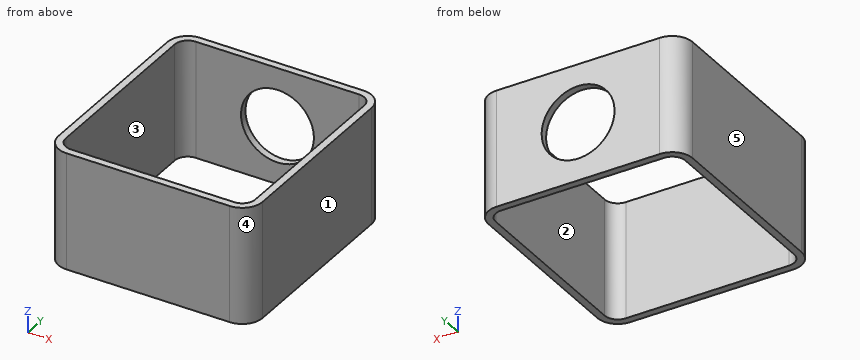
```python
from build123d import *

# Parameters (mm, degrees)
SKETCH_1_W          = 28
SKETCH_1_H          = 30
SKETCH_1_W_2        = 26
SKETCH_1_H_2        = 28
EXTRUDE_1_DEPTH     = 16
FILLET_1_R          = 1.8
FILLET_2_R          = 2.8
SKETCH_2_R          = 5
CUT_EXTRUDE_1_DEPTH = 16


with BuildPart() as part:
    # Эскиз1 → Бобышка-Вытянуть1 (new body)
    with BuildSketch(Plane.XY):
        with Locations((14, 15)):
            Rectangle(SKETCH_1_W, SKETCH_1_H)
        with Locations((14, 15)):
            Rectangle(SKETCH_1_W_2, SKETCH_1_H_2, mode=Mode.SUBTRACT)
    extrude(amount=EXTRUDE_1_DEPTH)

    # Скругление1
    fillet_1_edges = [part.edges().sort_by_distance(p)[0] for p in [
        (27, 29, 8),
        (1, 29, 8),
        (1, 1, 8),
        (27, 1, 8),
    ]]
    fillet(fillet_1_edges, radius=FILLET_1_R)

    # Скругление2
    fillet_2_edges = [part.edges().sort_by_distance(p)[0] for p in [
        (0, 30, 8),
        (28, 30, 8),
        (28, 0, 8),
        (0, 0, 8),
    ]]
    fillet(fillet_2_edges, radius=FILLET_2_R)

    # Эскиз2 → Вырез-Вытянуть1 (cut)
    with BuildSketch(Plane(origin=(0, 30, 0), x_dir=(1, 0, 0), z_dir=(0, 1, 0))):
        with Locations(Location((14, -8, 0), (0, 0, 270))):
            Circle(SKETCH_2_R)
    extrude(amount=-CUT_EXTRUDE_1_DEPTH, mode=Mode.SUBTRACT)


solid = part.part
```
Design review of the part built by this model. Coordinates are the model's own, in mm. Face numbers are marked on the shaded views. A direction names the side the tool comes from. Round coordinates to 2 decimals unless told otherwise and drop trailing zeros. Write each loop counter-clockwise with the first axis right and the second up, starting at its lowest first coordinate (ties: lowest second). Pieces come first, ordered by that corner, then holes. Notation, with made-up numbers: (-3.75, 46) -> (35.25, 46) arc R25 cw to (35.25, 62) -> close; hole circle Ø2 at (53, 23.25). An arc over 180 degrees is marked (long way). Write item = value, one per line. Start each with the question number.
1) Take a section at D-D, the plane z = 1.5. State the section outline as (x, y) points.
2) Mouldability with a two-part tool opening along X and no side actions: class the marked faces 3, 4 and 5 as +X half, -X half, draft (parallel to the pull), parting line (faces both ways), or undercut.
3) Take a section at A-A, the plane x = 10. State the section outline as (y, z) points.
4) Tool access review of the marked faces 1 and 2: name each direction out of +Z, -Z, +X, -X, +Y, -Y from which nothing blocks a thin tool from reaching the whole face with its end or side.
5) Take a section at B-B, the plane y = 8.25. State the section outline as (x, z) points, plus the area to 3 significant figures.
6) Take a section at C-C, the plane x = 6.75. State the section outline as (y, z) points.
7) Wall thickness on probe 1 along Y at (x, z) = (5, 12); probe 2 along X at (y, z) = (22, 14.75); probe 3 along X at (y, z) = (29.65, 8): over which ranges is each line inside the solid? List them lowest first. Write a range as from..to.
Results list:
q1.outline = (0, 2.8) arc R2.8 ccw to (2.8, 0) -> (25.2, 0) arc R2.8 ccw to (28, 2.8) -> (28, 27.2) arc R2.8 ccw to (25.2, 30) -> (2.8, 30) arc R2.8 ccw to (0, 27.2) -> close; hole (1, 2.8) arc R1.8 ccw to (2.8, 1) -> (25.2, 1) arc R1.8 ccw to (27, 2.8) -> (27, 27.2) arc R1.8 ccw to (25.2, 29) -> (2.8, 29) arc R1.8 ccw to (1, 27.2) -> close
q2.face_3 = undercut
q2.face_4 = +X half
q2.face_5 = -X half
q3.outline = (0, 0) -> (1, 0) -> (1, 16) -> (0, 16) -> close; (29, 0) -> (30, 0) -> (30, 5) -> (29, 5) -> close; (29, 11) -> (30, 11) -> (30, 16) -> (29, 16) -> close
q4.face_1 = +Z, -Z, +X, +Y, -Y
q4.face_2 = +Z, -Z
q5.outline = (0, 0) -> (1, 0) -> (1, 16) -> (0, 16) -> close; (27, 0) -> (28, 0) -> (28, 16) -> (27, 16) -> close
q5.area = 32.0 mm²
q6.outline = (0, 0) -> (1, 0) -> (1, 16) -> (0, 16) -> close; (29, 0) -> (30, 0) -> (30, 16) -> (29, 16) -> close
q7.probe_1 = 0..1, 29..30
q7.probe_2 = 0..1, 27..28
q7.probe_3 = 1.44..9, 19..26.56
